Geometry: final body of the model. Coordinates: model frame, mm. A direction names the side the tool comes from. Give positions to 0.01 mm unless a question says otherwise; leave off trailing zeros. Write each loop counter-clockwise with the first axis right and the second up, starting at its lowest first coordinate (ties: lowest second). Pieces come first, ordered by that corner, then holes.
```python
from build123d import *

# Parameters (mm, degrees)
MAIN_SHAPE_DEPTH        = 0.6
TABS_DEPTH              = 154.060061459
TABS_DEPTH_BACK         = 154.060061459
CHIN_GUARD_DEPTH        = 0.6
FILLET1_R               = 20
CUT_EXTRUDE1_DEPTH      = 172.662513141
CUT_EXTRUDE1_DEPTH_BACK = 172.662513141


with BuildPart() as part:
    # Sketch1 → Main Shape (new body)
    with BuildSketch(Plane.XY):
        with BuildLine():
            Line((-24, -91.764766734), (24, -91.764766734))
            Line((24, -91.764766734), (78.266232563, -84.05670244))
            ThreePointArc((78.266232563, -84.05670244), (97.655491519, -79.289252293), (115.711102551, -70.764766734))
            ThreePointArc((115.711102551, -70.764766734), (120.685143325, -65.658407438), (122.5, -58.764766734))
            ThreePointArc((122.5, -58.764766734), (120.227482046, -43.118277124), (113.597722286, -28.764766734))
            ThreePointArc((113.597722286, -28.764766734), (107.811505455, -22.955172168), (100.180351554, -19.955641477))
            Line((100.180351554, -19.955641477), (60.74391922, -13.264766734))
            ThreePointArc((60.74391922, -13.264766734), (50.804108255, -9.246591688), (43.461443341, -1.434367632))
            ThreePointArc((43.461443341, -1.434367632), (36.448172688, 5.805997675), (26.941855461, 9.15842781))
            Line((26.941855461, 9.15842781), (17, 10.235233266))
            Line((17, 10.235233266), (10, 0))
            Line((10, 0), (-10, 0))
            Line((-10, 0), (-17, 10.235233266))
            Line((-17, 10.235233266), (-26.941855461, 9.15842781))
            ThreePointArc((-26.941855461, 9.15842781), (-36.448172688, 5.805997675), (-43.461443341, -1.434367632))
            ThreePointArc((-43.461443341, -1.434367632), (-50.804108255, -9.246591688), (-60.74391922, -13.264766734))
            Line((-60.74391922, -13.264766734), (-100.180351554, -19.955641477))
            ThreePointArc((-100.180351554, -19.955641477), (-107.811505455, -22.955172168), (-113.597722286, -28.764766734))
            ThreePointArc((-113.597722286, -28.764766734), (-120.227482046, -43.118277124), (-122.5, -58.764766734))
            ThreePointArc((-122.5, -58.764766734), (-120.685143325, -65.658407438), (-115.711102551, -70.764766734))
            ThreePointArc((-115.711102551, -70.764766734), (-97.655491519, -79.289252293), (-78.266232563, -84.05670244))
            Line((-78.266232563, -84.05670244), (-24, -91.764766734))
        make_face()
    extrude(amount=MAIN_SHAPE_DEPTH)

    # Sketch2 → Tabs (cut, two sides: drawn at the far end of the back side and taken through both)
    with BuildSketch(Plane.XY.offset(0.6).offset(-TABS_DEPTH_BACK)):
        with BuildLine():
            Line((-121, -58.764766734), (-121, -56.764766734))
            Line((-121, -56.764766734), (-115.742268041, -53.771413729))
            ThreePointArc((-115.742268041, -53.771413729), (-113.511139955, -43.427720083), (-109.089826236, -33.814088314))
            Line((-109.089826236, -33.814088314), (-111.5, -28.264766734))
            Line((-111.5, -28.264766734), (-110.3, -26.664766734))
            Line((-110.3, -26.664766734), (-108.3, -25.664766734))
            Line((-108.3, -25.664766734), (-106.7, -26.864766734))
            Line((-106.7, -26.864766734), (-107.9, -28.464766734))
            Line((-107.9, -28.464766734), (-106.3, -29.664766734))
            Line((-106.3, -29.664766734), (-98.84870892, -19.729711961))
            Line((-98.84870892, -19.729711961), (-100.180351554, -19.955641477))
            ThreePointArc((-100.180351554, -19.955641477), (-107.811505455, -22.955172168), (-113.597722286, -28.764766734))
            ThreePointArc((-113.597722286, -28.764766734), (-120.227482046, -43.118277124), (-122.5, -58.764766734))
            ThreePointArc((-122.5, -58.764766734), (-120.767844146, -65.510135516), (-116, -70.586357152))
            Line((-116, -70.586357152), (-116, -58.764766734))
            Line((-116, -58.764766734), (-118, -58.764766734))
            Line((-118, -58.764766734), (-118, -60.764766734))
            Line((-118, -60.764766734), (-120, -60.764766734))
            Line((-120, -60.764766734), (-121, -58.764766734))
        make_face()
        with BuildLine():
            Line((110.3, -26.664766734), (111.5, -28.264766734))
            Line((111.5, -28.264766734), (109.089826236, -33.814088314))
            ThreePointArc((109.089826236, -33.814088314), (113.511139955, -43.427720083), (115.742268041, -53.771413729))
            Line((115.742268041, -53.771413729), (121, -56.764766734))
            Line((121, -56.764766734), (121, -58.764766734))
            Line((121, -58.764766734), (120, -60.764766734))
            Line((120, -60.764766734), (118, -60.764766734))
            Line((118, -60.764766734), (118, -58.764766734))
            Line((118, -58.764766734), (116, -58.764766734))
            Line((116, -58.764766734), (116, -70.586357152))
            ThreePointArc((116, -70.586357152), (120.767844146, -65.510135516), (122.5, -58.764766734))
            ThreePointArc((122.5, -58.764766734), (120.227482046, -43.118277124), (113.597722286, -28.764766734))
            ThreePointArc((113.597722286, -28.764766734), (107.811505455, -22.955172168), (100.180351554, -19.955641477))
            Line((100.180351554, -19.955641477), (98.84870892, -19.729711961))
            Line((98.84870892, -19.729711961), (106.3, -29.664766734))
            Line((106.3, -29.664766734), (107.9, -28.464766734))
            Line((107.9, -28.464766734), (106.7, -26.864766734))
            Line((106.7, -26.864766734), (108.3, -25.664766734))
            Line((108.3, -25.664766734), (110.3, -26.664766734))
        make_face()
    extrude(amount=TABS_DEPTH + TABS_DEPTH_BACK, mode=Mode.SUBTRACT)

    # Sketch5 → Chin guard (add)
    with BuildSketch(Plane.XY.offset(0.6)):
        Polygon((-78.266232563, -84.05670244), (-24, -121.764766734), (24, -121.764766734), (78.266232563, -84.05670244), (24, -91.764766734), (-24, -91.764766734), align=None)
    extrude(amount=-CHIN_GUARD_DEPTH)

    # Fillet1
    fillet1_edges = [part.edges().sort_by_distance(p)[0] for p in [
        (-24, -121.764766734, 0.3),
        (24, -121.764766734, 0.3),
        (78.266232563, -84.05670244, 0.3),
        (-78.266232563, -84.05670244, 0.3),
    ]]
    fillet(fillet1_edges, radius=FILLET1_R)

    # Sketch6 → Cut-Extrude1 (cut, two sides: drawn at the far end of the back side and taken through both)
    with BuildSketch(Plane.XY.offset(0.6).offset(-CUT_EXTRUDE1_DEPTH_BACK)):
        with BuildLine():
            Line((-60.74391922, -13.264766734), (-60.74391922, 16.735233266))
            Line((-60.74391922, 16.735233266), (60.74391922, 16.735233266))
            Line((60.74391922, 16.735233266), (60.74391922, -13.264766734))
            ThreePointArc((60.74391922, -13.264766734), (0, -8.148349205), (-60.74391922, -13.264766734))
        make_face()
    extrude(amount=CUT_EXTRUDE1_DEPTH + CUT_EXTRUDE1_DEPTH_BACK, mode=Mode.SUBTRACT)


solid = part.part
```
Item 1: Pull-direction query (X, two-part tool) for faces 4 (the face through (-102.63, -24.77, 0.3)), 5 (the face through (80.06, -16.54, 0.3)), 6 (the face through (0.85, -8.15, 0.3)); classes: +X half, -X half, draft (parallel to the pull), parting line (faces both ways), or undercut.
Found:
face 4: undercut
face 5: +X half
face 6: parting line
Item 2: Line query: L1, parallel to X at y = -28, z = 0.3; L2, parallel to Y at x = -4, z = 0.1; L3, parallel to Y at x = 107, z = 0.4. Output: solid intervals per line, ascending.
Found:
L1: x = -111.3 to -107.55, -105.05 to 105.05, 107.55 to 111.3
L2: y = -121.76 to -8.17
L3: y = -75.43 to -29.14, -27.26 to -26.64
Item 3: Reachability of faces 1 (the face through (102.5, -24.6, 0.3)), 2 (the face through (113.464, -43.287, 0.296)), 3 (the face through (-113.56, -43.57, 0.3)) from +Z, -Z, +X, -X, +Y, -Y: full face, straight path, thin tool, end or side. Return the list, or none.
Found:
face 1: +Z, -Z, +Y
face 2: +Z, -Z, +X
face 3: +Z, -Z, -X
Item 4: Pin query (flat end, axial travel): pin 1 Ø12 at (x, y) = (-88, -86) entering from +Z. Return the tip coordinate at first contact, or that it passes through.
Found:
pin 1: stops at z = 0.6
Item 5: Section B-B, the plane x = 96.5. Return the cut outline in (y, z), plus the area to 3 significant figures.
Found:
outline: (-79.69, 0) - (-19.33, 0) - (-19.33, 0.6) - (-79.69, 0.6) - close
area: 36.2 mm2
Item 6: Section A-A, the plane y = -76.5. Return the cut outline in (x, z), plus the area to 3 significant figures.
Found:
outline: (-104.66, 0) - (104.66, 0) - (104.66, 0.6) - (-104.66, 0.6) - close
area: 126 mm2
